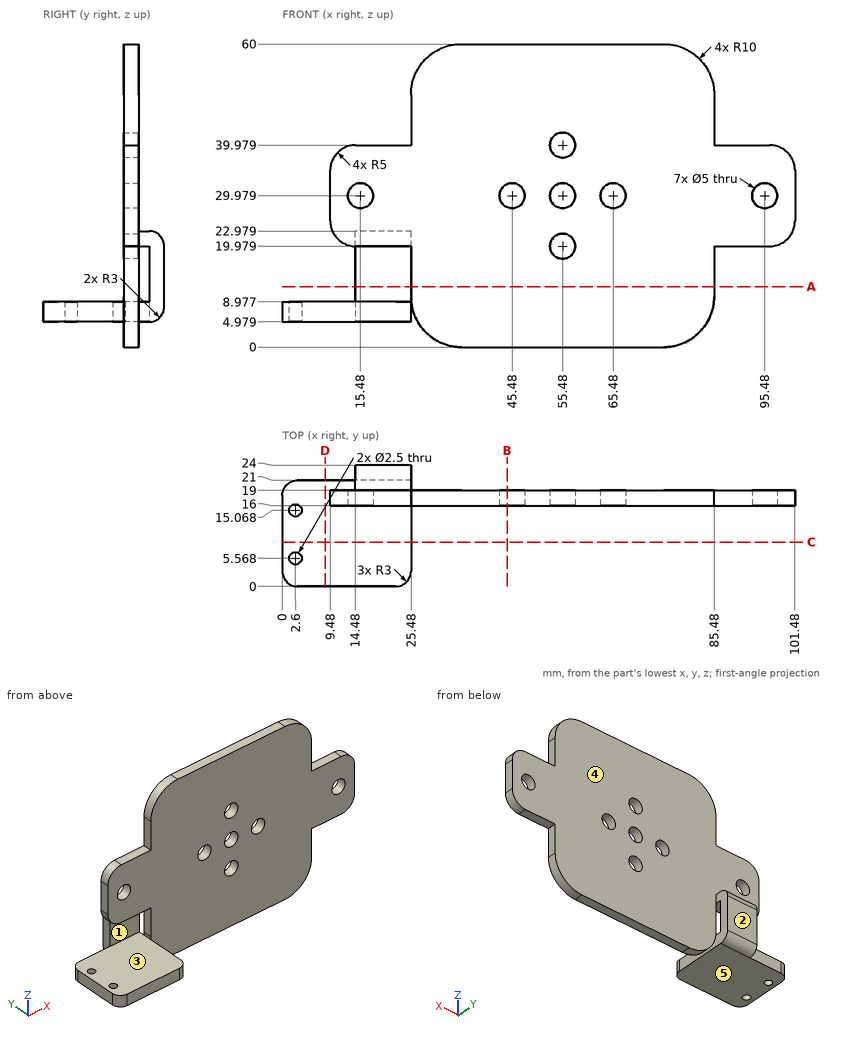
Answer from the drawing. Dimensions are ordinates in mm from the lowest x, y and z of the part. A direction names the side the tool comes from. Round coordinates to 2 decimals unless told otherwise and drop trailing zeros. Loops run counter-clockwise (first coordinate to the right, second up) from the corner with the lowest first, then second, coordinate; pieces in that order, holes last.
Q1. Each of these flat-tipped pins is pushed along its axis until it touches: pin 1 (4 mm diameter, centred on x = 65.48, z = 29.98, fed in from -Y); pin 2 (5 mm diameter, centred on x = 26.5, y = 13, fed in from -Z); pin 3 (2 mm diameter, centred on x = 20, y = 20.5, fed in from +Z); pin 4 (4.5 mm diameter, centred on x = 6.5, z = 7.5, fed in from +Y). Where does it stop, or does it pass through?
Q2. Section D-D on x = 8.5 is taken. Write down the section's boundary in (y, z).
Q3. Which of the six approach directions +Z, -Z, +X, -X, +Y, -Y give full straight-line access (tool end or side, diameter ignored) to the marked faces 1 and 2?
Q4. Determine the mould class of the marked faces 3, 4 and 5 for opening direction Z: released by +Z, released by -Z, zero draft, split by the parting line, or undercut.
Q5. Section A-A on z = 12 is taken. Write down the section's boundary in (x, y).
Q6. Consider probe 1 along Z at (x, y) = (18.5, 20.25); probe 2 along Y at (x, z) = (62, 29.5); probe 3 along Z at (x, y) = (5, 3.25). Determine where each line is inside the solid, lowest interval first.
Q7. Section B-B on x = 44.5 is taken. Write down the section's boundary in (y, z), and give its area (3 significant figures).
Q8. Section C-C on y = 8.75 is taken. Write down the section's boundary in (x, z), and give its area (3 significant figures).
Output:
1. pin 1: passes through
1. pin 2: stops at z = 4.98
1. pin 3: stops at z = 22.98
1. pin 4: stops at y = 21
2. outline: (0, 4.98) - (21, 4.98) - (21, 8.98) - (0, 8.98) - close
3. face 1: +X, -X, -Y
3. face 2: +Z, -Z, +X, -X, +Y
4. face 3: undercut
4. face 4: zero draft
4. face 5: released by -Z
5. outline: (14.48, 21) - (25.48, 21) - (25.48, 24) - (14.48, 24) - close; (25.48, 16) - (85.48, 16) - (85.48, 19) - (25.48, 19) - close
6. probe 1: z = 4.98 to 8.98, 19.98 to 22.98
6. probe 2: y = 16 to 19
6. probe 3: z = 4.98 to 8.98
7. outline: (16, 0) - (19, 0) - (19, 27.68) - (16, 27.68) - close; (16, 32.28) - (19, 32.28) - (19, 60) - (16, 60) - close
7. area: 166 mm2
8. outline: (0, 4.98) - (25.48, 4.98) - (25.48, 8.98) - (0, 8.98) - close
8. area: 102 mm2
